Autodesk Inventor part; units mm, degrees
ref_plane "YZ Plane" through (0, 0, 0) normal (1, 0, 0) x (0, 1, 0)
ref_plane "XZ Plane" through (0, 0, 0) normal (0, 1, 0) x (-1, 0, 0)
ref_plane "XY Plane" through (0, 0, 0) normal (0, 0, 1) x (1, 0, 0)
sketch "Sketch1" plane through (0, 0, 0) normal (0, 0, 1) x (1, 0, 0)
  line L0 (0, 0) -> (60, 0)
  line L1 (60, 0) -> (60, 3)
  line L2 (60, 3) -> (0, 3)
  line L3 (0, 3) -> (0, 0)
  dimension "d0" = 60
  dimension "d1" = 6
revolve "Revolution1" add sketch "Sketch1" angle 360 about axis through (0, 0, 0) along (1, 0, 0)
thread "Thread1"
chamfer "Chamfer1" distance 1 angle 45 2 edges at (0, -3, 0) (60, -3, 0)
sketch "Sketch2" plane through (0, 0, 0) normal (0, 0, 1) x (1, 0, 0)
  line L0 (1, 3) -> (59, 3)
  line L1 (60, 3) -> (50, 3)
  line L2 (50, 3) -> (50, 2)
  line L3 (50, 2) -> (60, 2)
  line L4 (60, 2) -> (60, 3)
  line L5 (60, -3) -> (60, 3)
  line L6 (60, -3) -> (50, -3)
  line L7 (50, -3) -> (50, -2)
  line L8 (50, -2) -> (60, -2)
  line L9 (60, -2) -> (60, -3)
  point P0 (0, 0)
  point P1 (50, 3)
  dimension "d8" = 4
  dimension "d15" = 10
extrude "Extrusion1" cut sketch "Sketch2" along normal through all both and the other way through all
sketch "Sketch3" plane through (50, -2, -2.2361) normal (0, -1, 0) x (1, 0, 0)
  circle A0 centre (7, 2.2361) radius 2
  line L0 (10, 2.2361) -> (10, 0.2361)
  point P0 (-50, 2.2361)
  dimension "d11" = 4
  dimension "d14" = 3
extrude "Extrusion2" cut sketch "Sketch3" against normal through all
properties part number "M6x1_THREADED_ROD_CPY_CPY"
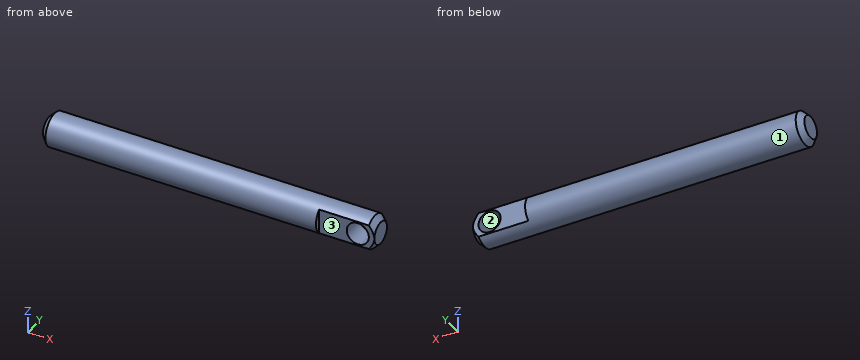
Read the model definition and answer for the solid it produces. Units are mm, in the model's axes. Face numbers are marked on the shaded views. Round coordinates to 2 decimals unless told otherwise and drop trailing zeros. Write each loop counter-clockwise with the first axis right and the second up, starting at its lowest first coordinate (ties: lowest second). Pieces come first, ordered by that corner, then holes. Notation, with made-up numbers: (48.25, 18) - (78.25, 18) arc R33 cw to (78.25, 54) - close; hole circle Ø8 at (62.25, 41). An arc over 180 degrees is marked (long way). Use a Markdown table: item, result.
(1) Each of these flat-tipped pins is pushed along its axis until it touches: pin 1 Ø0.8 at (y, z) = (-2.5, -1) entering from +X; pin 2 Ø3.5 at (x, z) = (53.5, -0.5) entering from -Y; pin 3 Ø3.5 at (x, z) = (57, 0) entering from +Y; pin 4 Ø2 at (x, z) = (47.5, -2) entering from +Y. Where does it stop, or does it pass through?
Reported:
| item | result |
|---|---|
| pin 1 | x = 50 |
| pin 2 | y = -2 |
| pin 3 | through |
| pin 4 | y = 2.83 |
(2) The part is cut by section C-C (x = 7). Write down the section's boundary in (y, z).
Reported:
| item | result |
|---|---|
| outline | circle Ø6 at (0, 0) |
(3) The part is cut by section A-A (y = 0). Write down the section's boundary in (x, z), then the cut area to 3 significant figures.
Reported:
| item | result |
|---|---|
| outline | (0, -2) - (1, -3) - (59, -3) - (60, -2) - (60, 2) - (59, 3) - (1, 3) - (0, 2) - close; hole circle Ø4 at (57, 0) |
| area | 345 mm2 |
(4) Straight lines are drawn through the part: line 1 along X through (y, z) = (0.95, 0.05); line 2 along X through (y, z) = (-1.3, 0.45); line 3 along Z through (x, y) = (57, -0.1). For each, find the intervals that lie inside material, in ascending order. Write a range as [from, to].
Reported:
| item | result |
|---|---|
| line 1 | [0, 55], [59, 60] |
| line 2 | [0, 55.05], [58.95, 60] |
| line 3 | [-3, -2], [2, 3] |
(5) The part is cut by section B-B (x = 57). Write down the section's boundary in (y, z), then the cut area to 3 significant figures.
Reported:
| item | result |
|---|---|
| outline | (-2, -2.24) arc R3 ccw to (2, -2.24) - (2, -2) - (-2, -2) - close; (-2, 2) - (2, 2) - (2, 2.24) arc R3 ccw to (-2, 2.24) - close |
| area | 6.08 mm2 |
(6) The mould has two halves that part along Z. Classify the marked faces 1, 2 and 3: released by +Z, released by -Z, zero draft, split by the parting line, or undercut.
Reported:
| item | result |
|---|---|
| face 1 | split by the parting line |
| face 2 | undercut |
| face 3 | zero draft |
